Input: part model. Units: mm. Frame: model coordinates. Face numbers are marked on the shaded views. A direction names the side the tool comes from. Round coordinates to 2 decimals unless told otherwise and drop trailing zeros. Order: outer loops, then holes, each group sorted by start corner. A loop starts at its lowest first (then second) coordinate and runs counter-clockwise, first axis right, second up.
Item 1: Reachability of the marked faces 5, 6 and 7 from +Z, -Z, +X, -X, +Y, -Y: full face, straight path, thin tool, end or side. Return the list, or none.
Item 2: Line query: L1, parallel to X at y = 8.5, z = -14.5; L2, parallel to Z at x = 33.5, y = -20; L3, parallel to X at y = 16, z = -22.5. Output: solid intervals per line, ascending.
Item 3: Cut plane A-A on z = -10.5. Output: boundary loops of the cut face in (x, y).
Item 4: Cut plane B-B on z = -24.5. Output: boundary loops of the cut face in (x, y).
Item 5: Cut plane C-C on y = -17.5. Give the number of separate pieces and of enclosed holes in the cut face, then the cut area to 3 significant figures.
Item 6: Mould query, pull axis X, two halves, no side actions, for the marked faces 1, 2, 3 and 4. Classes: released by +X, released by -X, zero draft, split by the parting line, or undercut.
Item 7: First-contact query: pin 1 (1.9 mm diameter, centred on x = -2, y = -15, fed in from +Z); pin 2 (8 mm diameter, centred on y = -10, z = 8.5, fed in from +X); pin 3 (2.5 mm diameter, centred on x = -2.5, y = -7, fed in from +Z); pin 4 (15 mm diameter, centred on x = 34.59, z = 25.4, fed in from +Y). Flat tips, straight axial feed; report the tip coordinate or a pass-through.
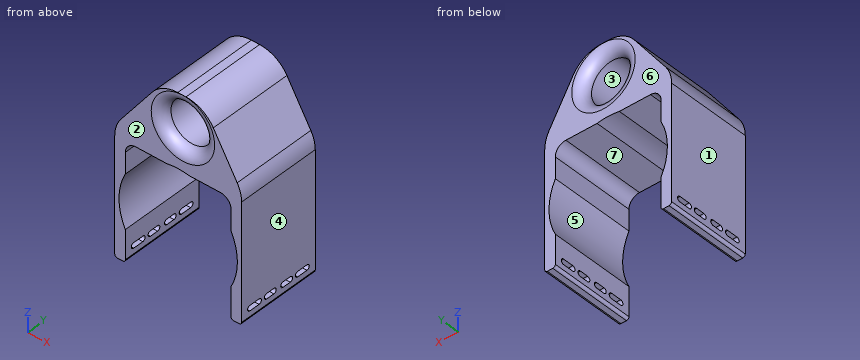
```python
from build123d import *

# Parameters (mm, degrees)
SKETCH1_R           = 12.7
BOSS_EXTRUDE1_DEPTH = 25.4
SKETCH2_R           = 35.56
CUT_EXTRUDE1_DEPTH  = 50.8
CUT_EXTRUDE2_DEPTH  = 127
FILLET1_R           = 6.35


with BuildPart() as part:
    # Sketch1 → Boss-Extrude1 (new, symmetric)
    with BuildSketch(Plane(origin=(0, 0, 0), x_dir=(1, 0, 0), z_dir=(0, 1, 0))):
        with BuildLine():
            Line((6.35, 0), (57.15, 0))
            ThreePointArc((57.15, 0), (61.640128061, 1.859871939), (63.5, 6.35))
            Line((63.5, 6.35), (63.5, 68.326))
            ThreePointArc((63.5, 68.326), (63.946369265, 69.403630735), (65.024, 69.85))
            Line((65.024, 69.85), (68.326, 69.85))
            ThreePointArc((68.326, 69.85), (69.403630735, 69.403630735), (69.85, 68.326))
            Line((69.85, 68.326), (69.85, -1.133947157))
            ThreePointArc((69.85, -1.133947157), (69.173698323, -6.16482282), (67.192812606, -10.83849222))
            Line((67.192812606, -10.83849222), (52.827309323, -35.104545063))
            ThreePointArc((52.827309323, -35.104545063), (45.869297101, -41.949532976), (36.434496717, -44.45))
            Line((36.434496717, -44.45), (31.486207829, -44.45))
            ThreePointArc((31.486207829, -44.45), (22.919370647, -42.415046303), (16.182781968, -36.744939705))
            Line((16.182781968, -36.744939705), (-2.603425861, -11.403832022))
            ThreePointArc((-2.603425861, -11.403832022), (-5.389123288, -6.032678275), (-6.35, -0.058892317))
            Line((-6.35, -0.058892317), (-6.35, 68.326))
            ThreePointArc((-6.35, 68.326), (-5.903630735, 69.403630735), (-4.826, 69.85))
            Line((-4.826, 69.85), (-1.524, 69.85))
            ThreePointArc((-1.524, 69.85), (-0.446369265, 69.403630735), (0, 68.326))
            Line((0, 68.326), (0, 6.35))
            ThreePointArc((0, 6.35), (1.859871939, 1.859871939), (6.35, 0))
        make_face()
        with Locations(Location((34.5948, -25.4, 0), (0, 0, 270))):
            Circle(SKETCH1_R, mode=Mode.SUBTRACT)
    extrude(amount=BOSS_EXTRUDE1_DEPTH, both=True)

    # Sketch2 → Cut-Extrude1 (cut)
    with BuildSketch(Plane(origin=(0, 25.4, 0), x_dir=(1, 0, 0), z_dir=(0, 1, 0))):
        with Locations((31.75, 34.925)):
            Circle(SKETCH2_R)
    extrude(amount=-CUT_EXTRUDE1_DEPTH, mode=Mode.SUBTRACT)

    # Sketch3 → Cut-Extrude2 (cut)
    with BuildSketch(Plane(origin=(69.85, 0, 0), x_dir=(0, 0, -1), z_dir=(1, 0, 0))):
        with BuildLine():
            Line((65.0875, -3.175), (65.0875, -8.149687283))
            ThreePointArc((65.0875, -8.149687283), (63.5, -9.737187283), (61.9125, -8.149687283))
            Line((61.9125, -8.149687283), (61.9125, -3.175))
            ThreePointArc((61.9125, -3.175), (63.5, -1.5875), (65.0875, -3.175))
        make_face()
        with BuildLine():
            Line((65.0875, -13.335), (65.0875, -19.685))
            ThreePointArc((65.0875, -19.685), (63.5, -21.2725), (61.9125, -19.685))
            Line((61.9125, -19.685), (61.9125, -13.335))
            ThreePointArc((61.9125, -13.335), (63.5, -11.7475), (65.0875, -13.335))
        make_face()
        with BuildLine():
            Line((65.0875, 13.335), (65.0875, 19.685))
            ThreePointArc((65.0875, 19.685), (63.5, 21.2725), (61.9125, 19.685))
            Line((61.9125, 19.685), (61.9125, 13.335))
            ThreePointArc((61.9125, 13.335), (63.5, 11.7475), (65.0875, 13.335))
        make_face()
        with BuildLine():
            Line((65.0875, 3.175), (65.0875, 8.149687283))
            ThreePointArc((65.0875, 8.149687283), (63.5, 9.737187283), (61.9125, 8.149687283))
            Line((61.9125, 8.149687283), (61.9125, 3.175))
            ThreePointArc((61.9125, 3.175), (63.5, 1.5875), (65.0875, 3.175))
        make_face()
    extrude(amount=-CUT_EXTRUDE2_DEPTH, mode=Mode.SUBTRACT)

    # Fillet1
    fillet1_edges = [part.edges().sort_by_distance(p)[0] for p in [
        (34.5948, -25.4, 12.7),
        (34.5948, 25.4, 12.7),
    ]]
    fillet(fillet1_edges, radius=FILLET1_R - 0.0001)  # a hair under: the kernel refuses the full size


solid = part.part
```
From the geometry:
1. face 5: +Y, -Y
1. face 6: +Z, -Z, +X, -X, +Y
1. face 7: -Z, +Y, -Y
2. L1: x = -6.35 to 0, 63.5 to 69.85
2. L2: z = 0.59 to 12.68, 38.12 to 44.45
2. L3: x = -6.35 to -1.57, 65.07 to 69.85
3. outline: (-6.35, -25.4) - (0, -25.4) - (0, 25.4) - (-6.35, 25.4) - close; (63.5, -25.4) - (69.85, -25.4) - (69.85, 25.4) - (63.5, 25.4) - close
4. outline: (-6.35, -25.4) - (-2.25, -25.4) - (-2.25, 25.4) - (-6.35, 25.4) - close; (65.75, -25.4) - (69.85, -25.4) - (69.85, 25.4) - (65.75, 25.4) - close
5. separate pieces: 3
5. enclosed holes: 1
5. area: 2,570 mm2
6. face 1: released by -X
6. face 2: zero draft
6. face 3: undercut
6. face 4: released by +X
7. pin 1: stops at z = 13.5
7. pin 2: stops at x = 69.55
7. pin 3: stops at z = 13.23
7. pin 4: passes through
